from build123d import *

# Parameters (mm, degrees)
SKETCH1_W             = 104.2416
SKETCH1_H             = 41.91
BOSS_EXTRUDE1_DEPTH   = 0.8636
F_4_40_TAPPED_HOLE1_D = 2.2606


with BuildPart() as part:
    # Sketch1 → Boss-Extrude1 (new, symmetric)
    with BuildSketch(Plane(origin=(0, 0, 0), x_dir=(1, 0, 0), z_dir=(0, 1, 0))):
        Rectangle(SKETCH1_W, SKETCH1_H)
    extrude(amount=BOSS_EXTRUDE1_DEPTH, both=True)

    # #4-40 Tapped Hole1 (through all)
    with Locations(Plane(origin=(0, 0.8636, 0), x_dir=(1, 0, 0), z_dir=(0, 1, 0))):
        with Locations((-48.3108, 17.145), (-36.8808, -15.875), (34.3408, 17.145), (36.8808, -13.335)):
            Hole(F_4_40_TAPPED_HOLE1_D / 2)


solid = part.part
Work out the finished part from the listing and answer in its coordinate system (mm). Round coordinates to 2 decimals unless told otherwise and drop trailing zeros.
1) The mould has two halves that part along Z. Classify faces 1 (the cylindrical face through (37.028, -0.012, 12.214)), 2 (the flat face through (-1, 0, -20.955)), 3 (the flat face through (-52.121, 0, 0)): pulls with the +Z half, pulls with the -Z half, needs draft (parallel to the pull), parting line crosses it, or undercut.
2) Given pin 1 Ø2.5 at (x, z) = (-48.31, -17.14) entering from +Y, flat-ended and moving along its own axis, determine where the tip first touches the part or whether it passes through.
3) Straight lines are drawn through the part: line 1 (Z direction, x = -37, y = -0.1) (3 decimals); line 2 (X direction, y = 0.15, z = 12.5); line 3 (X direction, y = 0.05, z = -18). For each, find the intervals that lie inside material, in ascending order.
Completed:
1. face 1: undercut
1. face 2: pulls with the -Z half
1. face 3: needs draft
2. pin 1: stops at y = 0.86
3. line 1: z = -20.955 to 14.751, 16.999 to 20.955
3. line 2: x = -52.12 to 36.12, 37.64 to 52.12
3. line 3: x = -52.12 to -49.05, -47.57 to 33.6, 35.08 to 52.12
